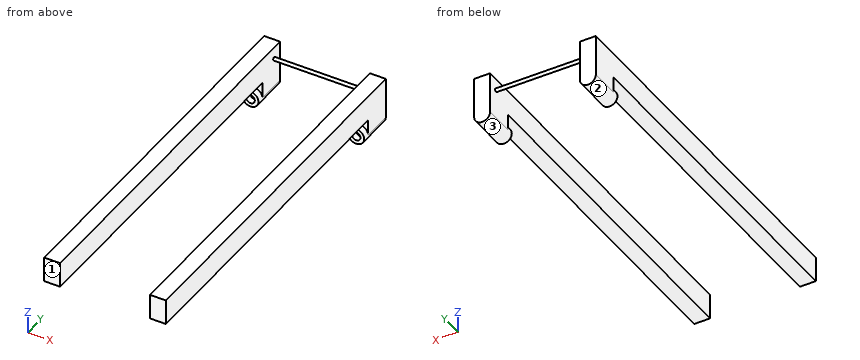
```python
from build123d import *

# Parameters (mm, degrees)
SKETCH1_R             = 60
SKETCH1_R_2           = 32.528667591
BOSS_EXTRUDE1_DEPTH   = 50
SKETCH1_R_3           = 31.696746535
BOSS_EXTRUDE1_2_DEPTH = 50
SKETCH2_R             = 60
BOSS_EXTRUDE2_DEPTH   = 225.5
SKETCH5_W             = 120
SKETCH5_H             = 225.5
BOSS_EXTRUDE3_DEPTH   = 310
SKETCH6_W             = 120
SKETCH6_H             = 190
BOSS_EXTRUDE4_DEPTH   = 2574.5
SKETCH7_W             = 190
SKETCH7_H             = 225.5
BOSS_EXTRUDE5_DEPTH   = 676
SKETCH9_W             = 190
SKETCH9_H             = 225.5
SKETCH9_R             = 12.5
CUT_EXTRUDE1_DEPTH    = 676


with BuildPart() as part:
    # Sketch1 → Boss-Extrude1 (new body)
    with BuildSketch(Plane(origin=(0, 0, 0), x_dir=(1, 0, 0), z_dir=(0, 1, 0))):
        with Locations(Location((-398, 0, 0), (0, 0, 270))):
            Circle(SKETCH1_R)
        with Locations(Location((-398, 0, 0), (0, 0, 270))):
            Circle(SKETCH1_R_2, mode=Mode.SUBTRACT)
    extrude(amount=BOSS_EXTRUDE1_DEPTH)



with BuildPart() as body_2:
    # Sketch1 → Boss-Extrude1 2 (new body)
    with BuildSketch(Plane(origin=(0, 0, 0), x_dir=(1, 0, 0), z_dir=(0, 1, 0))):
        with Locations(Location((398, 0, 0), (0, 0, 270))):
            Circle(SKETCH1_R)
        with Locations(Location((398, 0, 0), (0, 0, 270))):
            Circle(SKETCH1_R_3, mode=Mode.SUBTRACT)
    extrude(amount=BOSS_EXTRUDE1_2_DEPTH)


with BuildPart() as part_1:
    add(part.part)

    add(body_2.part)  # Boss-Extrude2 merges body 2
    # Sketch2 → Boss-Extrude2 (add)
    with BuildSketch(Plane(origin=(0, 50, 0), x_dir=(1, 0, 0), z_dir=(0, 1, 0))):
        with Locations(Location((398, 0, 0), (0, 0, 270))):
            Circle(SKETCH2_R)
        with Locations(Location((-398, 0, 0), (0, 0, 270))):
            Circle(SKETCH2_R)
    extrude(amount=BOSS_EXTRUDE2_DEPTH)

    # Sketch5 → Boss-Extrude3 (add)
    with BuildSketch(Plane.XY):
        with Locations((-398, 162.75)):
            Rectangle(SKETCH5_W, SKETCH5_H)
        with Locations((398, 162.75)):
            Rectangle(SKETCH5_W, SKETCH5_H)
    extrude(amount=BOSS_EXTRUDE3_DEPTH)

    # Sketch6 → Boss-Extrude4 (add)
    with BuildSketch(Plane.XZ.offset(-50)):
        with Locations((398, 215)):
            Rectangle(SKETCH6_W, SKETCH6_H)
        with Locations((-398, 215)):
            Rectangle(SKETCH6_W, SKETCH6_H)
    extrude(amount=BOSS_EXTRUDE4_DEPTH)

    # Sketch7 → Boss-Extrude5 (add)
    with BuildSketch(Plane(origin=(-338, 0, 0), x_dir=(0, 0, -1), z_dir=(1, 0, 0))):
        with Locations((-215, 162.75)):
            Rectangle(SKETCH7_W, SKETCH7_H)
    extrude(amount=BOSS_EXTRUDE5_DEPTH)

    # Sketch9 → Cut-Extrude1 (cut)
    with BuildSketch(Plane.ZY.offset(-338)):
        with Locations((215, 162.75)):
            Rectangle(SKETCH9_W, SKETCH9_H)
        with Locations((220, 200.5)):
            Circle(SKETCH9_R, mode=Mode.SUBTRACT)
    extrude(amount=CUT_EXTRUDE1_DEPTH, mode=Mode.SUBTRACT)


solid = part_1.part
```
The listing builds one solid part. Answer for the finished solid, in the listing's coordinates (mm). Face numbers are marked on the shaded views. Coordinates: 2 decimals unless noted, no trailing zeros. Write each loop counter-clockwise with the first axis right and the second up, starting at its lowest first coordinate (ties: lowest second). Pieces come first, ordered by that corner, then holes. Notation, with made-up numbers: (61, 47) - (109, 47) arc R23 cw to (109, 60) - close; hole circle Ø1 at (7.5, 87.25). An arc over 180 degrees is marked (long way). Return JSON: item names as keys, results as strings. Group by question number.
Q1. For a pull along Z with two mould halves and no side action, classify the marked faces 1, 2 and 3 as +Z half, -Z half, draft (parallel to the pull), parting line (faces both ways), or undercut.
Q2. The part is cut by section A-A on y = -132.5. Write down the section's boundary in (x, z).
Q3. The part is cut by section B-B on x = 398. Write down the section's boundary in (y, z), and give its area (3 significant figures).
Q4. The part is cut by section C-C on x = 255. Write down the section's boundary in (y, z).
Q5. Find the intervals of material crossed by line 1 along X through (y, z) = (11.5, 0); line 2 along X through (y, z) = (-1726.5, 238.5); line 3 along Z through (x, y) = (380, -2221.5), in increasing order. Write a range as [from, to].
Evaluation:
{
 "1": {"face 1": "draft", "face 2": "undercut", "face 3": "undercut"},
 "2": {"outline": "(-458, 120) - (-338, 120) - (-338, 310) - (-458, 310) - close; (338, 120) - (458, 120) - (458, 310) - (338, 310) - close"},
 "3": {"outline": "(-2524.5, 120) - (50, 120) - (50, 60) - (0, 60) - (0, 31.7) - (50, 31.7) - (50, -31.7) - (0, -31.7) - (0, -60) - (275.5, -60) - (275.5, 310) - (-2524.5, 310) - close", "area": "575,000 mm2"},
 "4": {"outline": "circle Ø25 at (200.5, 220)"},
 "5": {"line 1": "x = [-458, -430.53], [-365.47, -338], [338, 366.3], [429.7, 458]", "line 2": "x = [-458, -338], [338, 458]", "line 3": "z = [120, 310]"}
}
